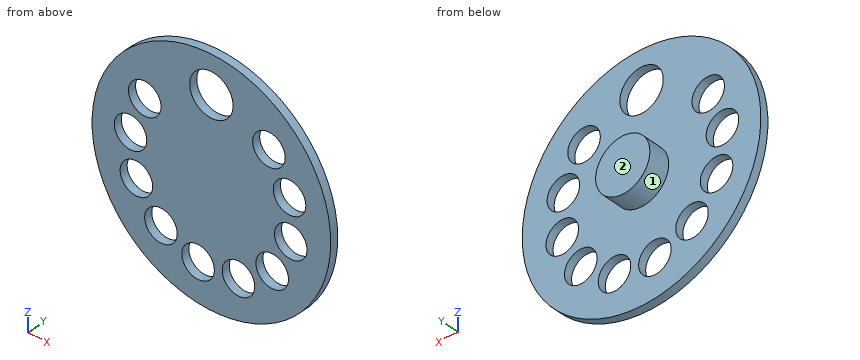
```python
from build123d import *

# Parameters (mm, degrees)
F0_R     = 22
F0_R_2   = 3
F0_R_3   = 4
F1_DEPTH = 1.5
F2_R     = 5
F3_DEPTH = 4


with BuildPart() as f1:
    # F0 (on Front) → F1 (new body)
    with BuildSketch(Plane.XZ):
        Circle(F0_R)
        with Locations((-9.303532, -11.766235)):
            Circle(F0_R_2, mode=Mode.SUBTRACT)
        with Locations((-2.461368, -14.796678)):
            Circle(F0_R_2, mode=Mode.SUBTRACT)
        with Locations((-13.830201, -5.80737)):
            Circle(F0_R_2, mode=Mode.SUBTRACT)
        with Locations((4.99339, -14.144471)):
            Circle(F0_R_2, mode=Mode.SUBTRACT)
        with Locations((11.205376, -9.971938)):
            Circle(F0_R_2, mode=Mode.SUBTRACT)
        with Locations((14.628528, -3.317554)):
            Circle(F0_R_2, mode=Mode.SUBTRACT)
        with Locations((-14.91476, 1.596853)):
            Circle(F0_R_2, mode=Mode.SUBTRACT)
        with Locations((-12.287281, 8.603647)):
            Circle(F0_R_2, mode=Mode.SUBTRACT)
        with Locations((10.606602, 10.606602)):
            Circle(F0_R_2, mode=Mode.SUBTRACT)
        with Locations((14.41088, 4.162515)):
            Circle(F0_R_2, mode=Mode.SUBTRACT)
        with Locations((0, 15)):
            Circle(F0_R_3, mode=Mode.SUBTRACT)
    extrude(amount=F1_DEPTH)

    # F2 (on face) → F3 (join)
    with BuildSketch(Plane(origin=(0, 0, 0), x_dir=(-1, 0, 0), z_dir=(0, 1, 0))):
        Circle(F2_R)
    extrude(amount=F3_DEPTH)


solid = f1.part
```
The model under review builds one solid part; all positions refer to its coordinate system, in mm. Face numbers are marked on the shaded views. A direction names the side the tool comes from. Round coordinates to 2 decimals unless told otherwise and drop trailing zeros. Order: outer loops, then holes, each group sorted by start corner. A loop starts at its lowest first (then second) coordinate and runs counter-clockwise, first axis right, second up. Notation, with made-up numbers: (50, -39.75) -> (85, -39.75) arc R30 cw to (85, -10.75) -> close; hole circle Ø9 at (-20, 50.25). An arc over 180 degrees is marked (long way). Use a Markdown table: item, result.
Q1. We need section A-A on x = 0. Write out the cut boundary in (y, z).
Values:
| item | result |
|---|---|
| outline | (-1.5, -22) -> (0, -22) -> (0, -16.51) -> (-1.5, -16.51) -> close; (-1.5, -13.08) -> (0, -13.08) -> (0, -5) -> (4, -5) -> (4, 5) -> (0, 5) -> (0, 11) -> (-1.5, 11) -> close; (-1.5, 19) -> (0, 19) -> (0, 22) -> (-1.5, 22) -> close |
Q2. We need section B-B on z = 17.5. Write out the cut boundary in (x, y), then the cut area to 3 significant figures.
Values:
| item | result |
|---|---|
| outline | (-13.33, -1.5) -> (-3.12, -1.5) -> (-3.12, 0) -> (-13.33, 0) -> close; (3.12, -1.5) -> (13.33, -1.5) -> (13.33, 0) -> (3.12, 0) -> close |
| area | 30.6 mm^2 |
Q3. Clearance check with flat-ended pins moving along their axes: P1, Ø5, axis at x = -9.3, z = -11.77, coming from the -Y side; P2, Ø8, axis at x = 14.41, z = 4.16, coming from the +Y side; P3, Ø1.5, axis at x = -3.5, y = 0.5, coming from the +Z side. State where each tip first meets the part, or that it passes through.
Values:
| item | result |
|---|---|
| P1 | passes through |
| P2 | stops at y = 0 |
| P3 | stops at z = 21.8 |
Q4. For line 1 (X direction, y = -0.1, z = -15); line 2 (Z direction, x = 0, y = -0.5); line 3 (X direction, y = -0.1, z = -10), list the stretches that pass through material, from the lowest coordinate up.
Values:
| item | result |
|---|---|
| line 1 | x = -16.09 to -5.45, 0.53 to 2.12, 7.87 to 16.09 |
| line 2 | z = -22 to -16.51, -13.08 to 11, 19 to 22 |
| line 3 | x = -19.6 to -11.73, -6.88 to 8.21, 14.21 to 19.6 |
Q5. We need section D-D on z = 3. Write out the cut boundary in (x, y), then the cut area to 3 significant figures.
Values:
| item | result |
|---|---|
| outline | (-21.79, -1.5) -> (-17.57, -1.5) -> (-17.57, 0) -> (-21.79, 0) -> close; (-12.26, -1.5) -> (11.65, -1.5) -> (11.65, 0) -> (4, 0) -> (4, 4) -> (-4, 4) -> (-4, 0) -> (-12.26, 0) -> close; (17.18, -1.5) -> (21.79, -1.5) -> (21.79, 0) -> (17.18, 0) -> close |
| area | 81.1 mm^2 |
Q6. We need section C-C on x = 6.5. Write out the cut boundary in (y, z).
Values:
| item | result |
|---|---|
| outline | (-1.5, -21.02) -> (0, -21.02) -> (0, -16.74) -> (-1.5, -16.74) -> close; (-1.5, -11.55) -> (0, -11.55) -> (0, 21.02) -> (-1.5, 21.02) -> close |
Q7. Tool access review of the marked faces 1 and 2: name each direction out of +Z, -Z, +X, -X, +Y, -Y from which nothing blocks a thin tool from reaching the whole face with its end or side.
Values:
| item | result |
|---|---|
| face 1 | +Y |
| face 2 | +Z, -Z, +X, -X, +Y |
